Here's the drawing with two shaded views (mm, measured from the low corner). I have some questions. A direction names the side the tool comes from. Give positions to 0.01 mm unless a question says otherwise; leave off trailing zeros. Write each loop counter-clockwise with the first axis right and the second up, starting at its lowest first coordinate (ties: lowest second). Pieces come first, ordered by that corner, then holes.
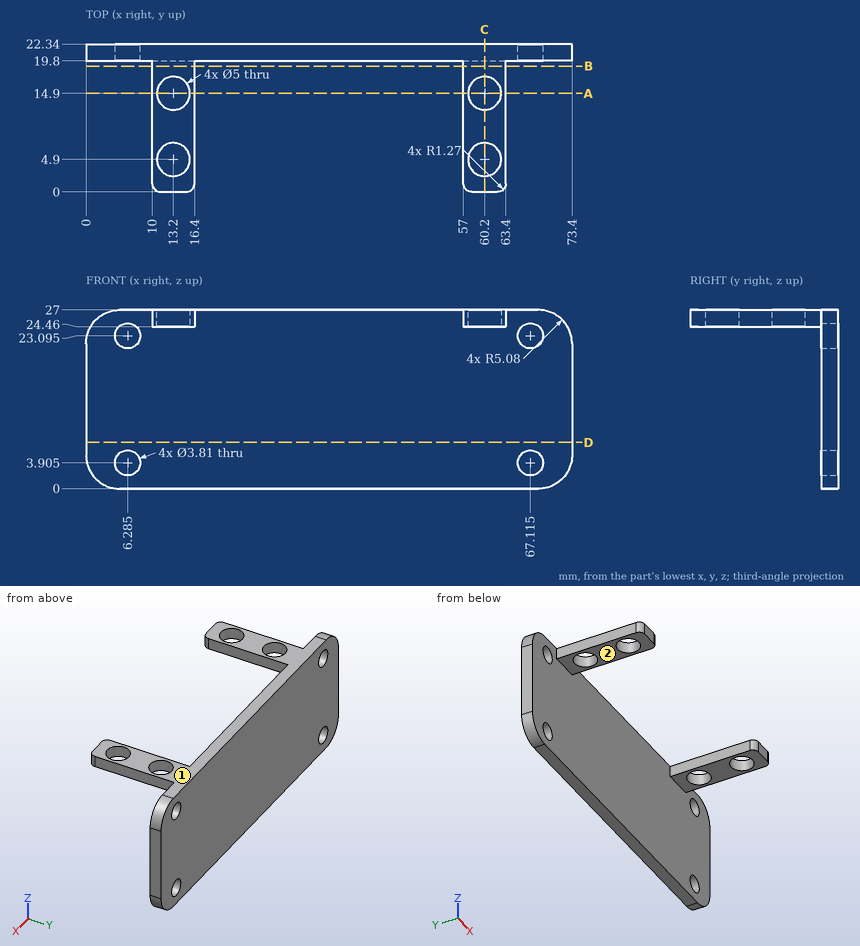
(1) For the marked faces 1 and 2, which set-ups out of +Z, -Z, +X, -X, +Y, -Y let a thin tool reach every point of the face, with its end or its side?
Returned:
face 1: +Z, +X, -X, +Y, -Y
face 2: -Z, +X, -X, -Y
(2) Imagine slicing it at A-A, the plane y = 14.9. Write out the boundary of the cut face in (x, z).
Returned:
outline: (10, 24.46) - (10.7, 24.46) - (10.7, 27) - (10, 27) - close; (15.7, 24.46) - (16.4, 24.46) - (16.4, 27) - (15.7, 27) - close; (57, 24.46) - (57.7, 24.46) - (57.7, 27) - (57, 27) - close; (62.7, 24.46) - (63.4, 24.46) - (63.4, 27) - (62.7, 27) - close
(3) Will these pins go through, and if not, where does the flat tip stop? P1, Ø12, axis at x = 17, y = 9.5, coming from the -Z side; P2, Ø0.8, axis at y = 10.5, z = 25.5, coming from the +X side; P3, Ø8, axis at x = 20.5, z = 4.5, coming from the -Y side.
Returned:
P1: stops at z = 24.46
P2: stops at x = 63.4
P3: stops at y = 19.8
(4) If I drill on L1, parallel to Y at x = 13.2, z = 26; L2, parallel to X at y = 10.5, z = 25.5; L3, parallel to Y at x = 63.5, z = 6.25, over which ranges is the centre line in solid material (lowest first)?
Returned:
L1: y = 0 to 2.4, 7.4 to 12.4, 17.4 to 22.34
L2: x = 10 to 16.4, 57 to 63.4
L3: y = 19.8 to 22.34
(5) Imagine slicing it at B-B, the plane y = 19. Write out the boundary of the cut face in (x, z), plus the area to 3 significant figures.
Returned:
outline: (10, 24.46) - (16.4, 24.46) - (16.4, 27) - (10, 27) - close; (57, 24.46) - (63.4, 24.46) - (63.4, 27) - (57, 27) - close
area: 32.5 mm2
(6) Imagine slicing it at D-D, the plane z = 7. Write out the boundary of the cut face in (x, y).
Returned:
outline: (0, 19.8) - (73.4, 19.8) - (73.4, 22.34) - (0, 22.34) - close
(7) Imagine slicing it at C-C, the plane x = 60.2. Write out the boundary of the cut face in (y, z).
Returned:
outline: (0, 24.46) - (2.4, 24.46) - (2.4, 27) - (0, 27) - close; (7.4, 24.46) - (12.4, 24.46) - (12.4, 27) - (7.4, 27) - close; (17.4, 24.46) - (19.8, 24.46) - (19.8, 0) - (22.34, 0) - (22.34, 27) - (17.4, 27) - close
